For this review, take the finished solid that the model builds, in its own axes (mm). Round coordinates to 2 decimals unless told otherwise and drop trailing zeros. Order: outer loops, then holes, each group sorted by start corner. A loop starts at its lowest first (then second) coordinate and runs counter-clockwise, first axis right, second up. Notation, with made-up numbers: (80.25, 87.25) - (134.25, 87.25) arc R33 ccw to (134.25, 126.25) - close; hole circle Ø3 at (3, 63). An arc over 180 degrees is marked (long way). One line per item, written item: value.
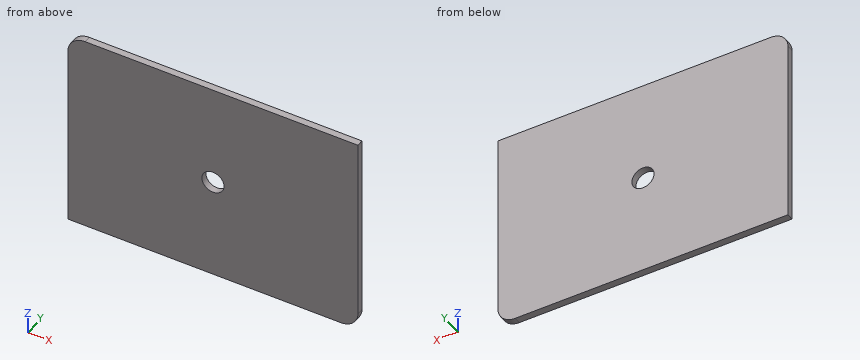
```python
from build123d import *

# Parameters (mm, degrees)
BOSS_EXTRUDE1_DEPTH = 4
CUT_EXTRUDE1_REACH  = 106.12
SKETCH3_R           = 6.5


with BuildPart() as part:
    # Sketch2 → Boss-Extrude1 (new body)
    with BuildSketch(Plane(origin=(0, 0, 0), x_dir=(1, 0, 0), z_dir=(0, 1, 0))):
        with BuildLine():
            Line((75, 60), (-85, 60))
            Line((-85, 60), (-85, -50))
            ThreePointArc((-85, -50), (-82.071067812, -57.071067812), (-75, -60))
            Line((-75, -60), (85, -60))
            Line((85, -60), (85, 50))
            ThreePointArc((85, 50), (82.071067812, 57.071067812), (75, 60))
        make_face()
    extrude(amount=-BOSS_EXTRUDE1_DEPTH)

    # Sketch3 → Cut-Extrude1 (cut, up to next)
    with BuildSketch(Plane(origin=(0, 0, 0), x_dir=(1, 0, 0), z_dir=(0, 1, 0)), mode=Mode.PRIVATE) as cut_extrude1_sk1:
        with Locations(Location((0, 0, 0), (0, 0, 270))):
            Circle(SKETCH3_R)
    cut_extrude1_tool1 = extrude(cut_extrude1_sk1.sketch, amount=-CUT_EXTRUDE1_REACH, mode=Mode.PRIVATE) & part.part
    add(cut_extrude1_tool1.solids().sort_by_distance((0, 0, 0))[0], mode=Mode.SUBTRACT)


solid = part.part
```
Item 1: Take a section at B-B (z = 0). Write out the cut boundary in (x, y), plus the area to 3 significant figures.
Returned:
outline: (-85, -4) - (-6.5, -4) - (-6.5, 0) - (-85, 0) - close; (6.5, -4) - (85, -4) - (85, 0) - (6.5, 0) - close
area: 628 mm^2
Item 2: Take a section at A-A (x = 0). Write out the cut boundary in (y, z), plus the area to 3 significant figures.
Returned:
outline: (-4, -60) - (0, -60) - (0, -6.5) - (-4, -6.5) - close; (-4, 6.5) - (0, 6.5) - (0, 60) - (-4, 60) - close
area: 428 mm^2
Item 3: Wall thickness on line 1 (X direction, y = -3.1, z = 0); line 2 (Z direction, x = 3, y = -1.1); line 3 (Z direction, x = 4.5, y = -0.45): over which ranges is each line inside the solid? List them lowest first.
Returned:
line 1: -85 to -6.5, 6.5 to 85
line 2: -60 to -5.77, 5.77 to 60
line 3: -60 to -4.69, 4.69 to 60
